Geometry check sheet. Reference: the model listing, model coordinates, mm. Round coordinates to 2 decimals unless told otherwise and drop trailing zeros. Order: outer loops, then holes, each group sorted by start corner. A loop starts at its lowest first (then second) coordinate and runs counter-clockwise, first axis right, second up.
(1) Sectioned sample at D-D (z = -172.5). Record the boundary of the cut face in (x, y), plus the area to 3 significant figures.
(2) Sectioned sample at C-C (x = -295.5). Record the boundary of the cut face in (y, z).
(3) Material ranges on line 1 along Z through (x, y) = (-505, -1.5); line 2 along X through (y, z) = (-4, 62.5); line 3 along X through (y, z) = (3.75, -416), recorded low to high.
(4) Sectioned sample at A-A (z = -357). Record the boundary of the cut face in (x, y), plus the area to 3 significant figures.
(5) Sectioned sample at B-B (y = 2). Record the boundary of the cut face in (x, z) (3 decimals), plus the area to 3 significant figures.
(6) Go/stop test with flat-tipped pins: pin 1 (1.5 mm diameter, centred on y = 0.5, z = -412.5, fed in from -X); pin 2 (4 mm diameter, centred on y = -4, z = -159, fed in from -X). Record where each tip stops, or that it passes through.
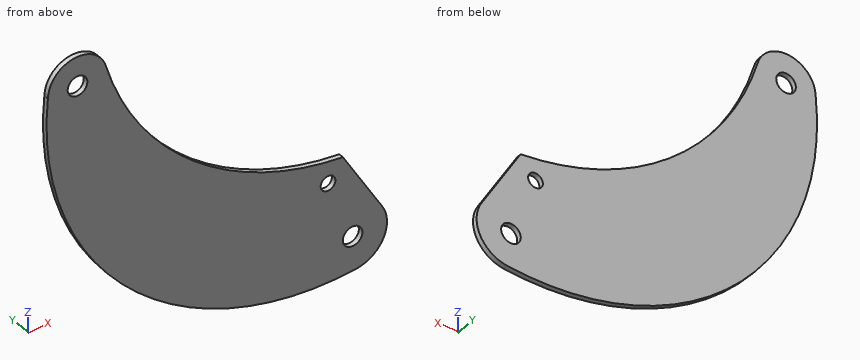
from build123d import *

# Parameters (mm, degrees)
SKETCH1_R           = 20
SKETCH1_R_2         = 15
BOSS_EXTRUDE1_DEPTH = 5


with BuildPart() as part:
    # Sketch1 → Boss-Extrude1 (new, symmetric)
    with BuildSketch(Plane(origin=(0, 0, 0), x_dir=(1, 0, 0), z_dir=(0, 1, 0))):
        with BuildLine():
            ThreePointArc((64.266544208, 563.161560744), (-397.988377373, 403.591852842), (-564.00499401, -56.38704581))
            Line((-564.00499401, -56.38704581), (-563.670163319, -56.38704581))
            ThreePointArc((-563.670163319, -56.38704581), (-563.576965484, -59.729956873), (-563.297661506, -63.062482866))
            ThreePointArc((-563.297661506, -63.062482866), (-508.728959827, -116.173403601), (-446.012064302, -72.986552362))
            ThreePointArc((-446.012064302, -72.986552362), (-266.335078189, 200.056876387), (36.550244036, 322.926786868))
            Line((36.550244036, 322.926786868), (116.550244036, 457.926786868))
            ThreePointArc((116.550244036, 457.926786868), (119.01905015, 524.75878079), (64.266544208, 563.161560744))
        make_face()
        with Locations(Location((-503.670163319, -56.38704581, 0), (0, 0, 270))):
            Circle(SKETCH1_R, mode=Mode.SUBTRACT)
        with Locations(Location((6.329836681, 363.61295419, 0), (0, 0, 270))):
            Circle(SKETCH1_R_2, mode=Mode.SUBTRACT)
        with Locations(Location((56.329836681, 493.61295419, 0), (0, 0, 270))):
            Circle(SKETCH1_R, mode=Mode.SUBTRACT)
    extrude(amount=BOSS_EXTRUDE1_DEPTH, both=True)


solid = part.part
Answer below:
1. outline: (-539.93, -5) - (-297.45, -5) - (-297.45, 5) - (-539.93, 5) - close
1. area: 2,420 mm2
2. outline: (-5, -483.7) - (5, -483.7) - (5, -174.35) - (-5, -174.35) - close
3. line 1: z = -257.4 to 36.43, 76.34 to 116.37
3. line 2: x = -563.36 to -522.71, -484.63 to -442.88
3. line 3: x = -385 to 91.7
4. outline: (-440.26, -5) - (-7.13, -5) - (-7.13, 5) - (-440.26, 5) - close; (19.79, -5) - (56.74, -5) - (56.74, 5) - (19.79, 5) - close
4. area: 4,700 mm2
5. outline: (-564.005, 56.387) arc R566.817 ccw to (64.267, -563.162) arc R70 ccw to (116.55, -457.927) - (36.55, -322.927) arc R550 cw to (-446.012, 72.987) arc R60 ccw to (-563.67, 56.387) - close; hole circle Ø40 at (-503.67, 56.387); hole circle Ø30 at (6.33, -363.613); hole circle Ø40 at (56.33, -493.613)
5. area: 194,000 mm2
6. pin 1: stops at x = -389.54
6. pin 2: stops at x = -544.64
